For this review, use the dimensioned drawing (mm, ordinates from the lowest corner) and the shaded views. A direction names the side the tool comes from. Round coordinates to 2 decimals unless told otherwise and drop trailing zeros. Loops run counter-clockwise (first coordinate to the right, second up) from the corner with the lowest first, then second, coordinate; pieces in that order, holes last. Notation, with made-up numbers: (26, 45) -> (70, 45) arc R22 ccw to (70, 59) -> close; hole circle Ø7 at (35.25, -23). An arc over 180 degrees is marked (long way). Write each question's results on one line, items separated by ' | '.
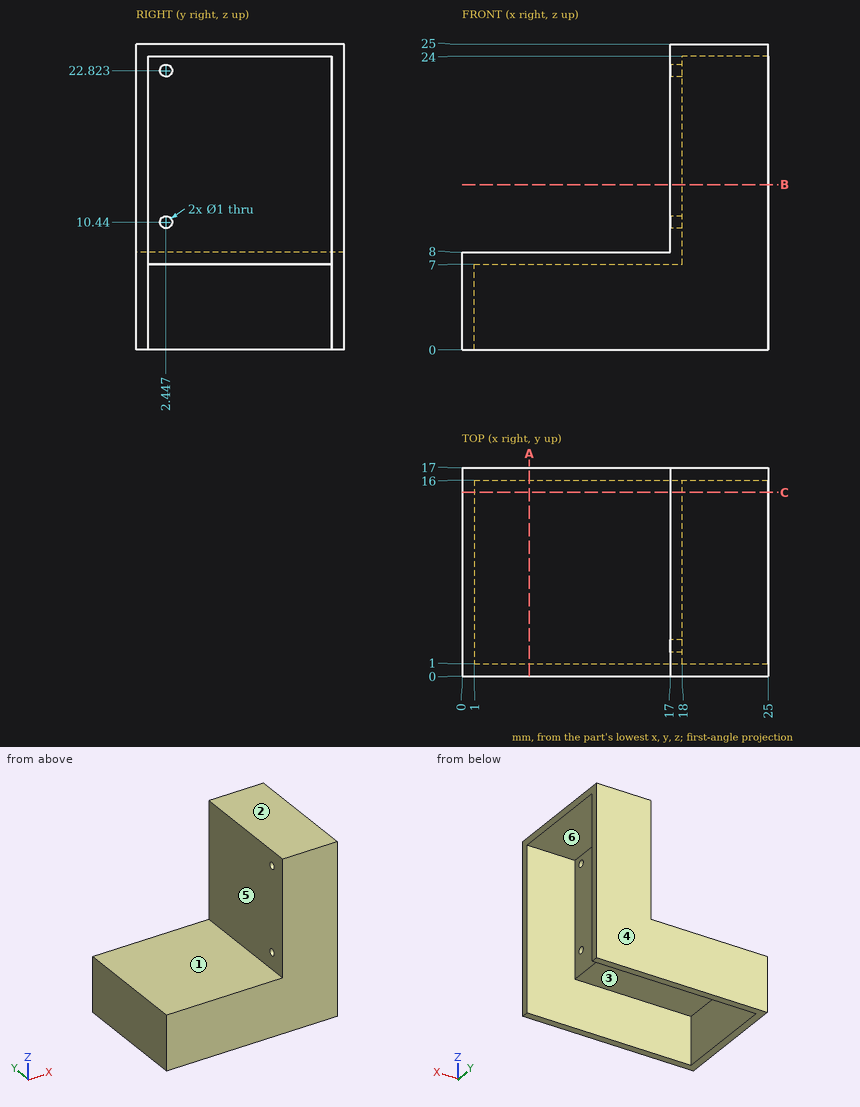
1. Tool access review of the marked faces 1, 2 and 3: name each direction out of +Z, -Z, +X, -X, +Y, -Y from which nothing blocks a thin tool from reaching the whole face with its end or side.
Values found:
face 1: +Z, -X, +Y, -Y | face 2: +Z, +X, -X, +Y, -Y | face 3: -Z, +X
2. Consider section C-C (y = 15). State the section outline as (x, z) points.
Values found:
outline: (0, 0) -> (1, 0) -> (1, 7) -> (18, 7) -> (18, 24) -> (25, 24) -> (25, 25) -> (17, 25) -> (17, 8) -> (0, 8) -> close
3. Consider section B-B (z = 13.5). State the section outline as (x, y) points.
Values found:
outline: (17, 0) -> (25, 0) -> (25, 1) -> (18, 1) -> (18, 16) -> (25, 16) -> (25, 17) -> (17, 17) -> close
4. For pin 1 (8 mm diameter, centred on y = 6.5, z = 9.5, fed in from -X); pin 2 (1 mm diameter, centred on y = 8, z = 14, fed in from -X); pin 3 (5.5 mm diameter, centred on y = 5, z = 2.5, fed in from +X); pin 4 (3 mm diameter, centred on x = 9.5, y = 4, fed in from +Z), all flat-tipped, find the tip position at first contact; note any pin that passes through.
Values found:
pin 1: stops at x = 0 | pin 2: stops at x = 17 | pin 3: stops at x = 1 | pin 4: stops at z = 8
5. To check wall thickness, follow probe 1 along Y at (x, z) = (23.5, 7); probe 2 along Z at (x, y) = (12.5, 1.25); probe 3 along X at (y, z) = (7.25, 9). State the ranges of each line that lie inside material, in increasing order.
Values found:
probe 1: y = 0 to 1, 16 to 17 | probe 2: z = 7 to 8 | probe 3: x = 17 to 18
6. Consider section A-A (x = 5.5). State the section outline as (y, z) points.
Values found:
outline: (0, 0) -> (1, 0) -> (1, 7) -> (16, 7) -> (16, 0) -> (17, 0) -> (17, 8) -> (0, 8) -> close
7. Draft analysis for pull direction Y (two halves, no side actions). For the marked faces 4, 5 and 6, state which applies: released by +Y, released by -Y, zero draft, split by the parting line, or undercut.
Values found:
face 4: released by +Y | face 5: zero draft | face 6: undercut
